from build123d import *

# Parameters (mm, degrees)
FILLET1_R     = 1
CHAMFER1_SIZE = 0.5
CHAMFER2_SIZE = 0.2


with BuildPart() as part:
    # Sketch1 → Revolve1 (revolve)
    with BuildSketch(Plane.XY, mode=Mode.PRIVATE) as revolve1_sk:
        Polygon((0, 0), (0, 8), (2.75, 8), (2.75, 6), (1.5, 6), (1.5, 0), align=None)
    revolve(revolve1_sk.sketch.rotate(Axis((0, 0, 0), (0, 1, 0)), 90), axis=Axis((0, 0, 0), (0, 1, 0)))

    # Fillet1
    fillet1_edges = [part.edges().sort_by_distance(p)[0] for p in [
        (0, 8, 2.75),
    ]]
    fillet(fillet1_edges, radius=FILLET1_R)

    # Chamfer1
    chamfer1_edges = [part.edges().sort_by_distance(p)[0] for p in [
        (0, 0, 1.5),
    ]]
    chamfer(chamfer1_edges, length=CHAMFER1_SIZE)

    # Chamfer2
    chamfer2_edges = [part.edges().sort_by_distance(p)[0] for p in [
        (0, 6, 2.75),
    ]]
    chamfer(chamfer2_edges, length=CHAMFER2_SIZE)


solid = part.part
Model file for the job. Use its own axes, mm. A direction names the side the tool comes from. Give positions to 0.01 mm unless a question says otherwise; leave off trailing zeros. Write each loop counter-clockwise with the first axis right and the second up, starting at its lowest first coordinate (ties: lowest second). Pieces come first, ordered by that corner, then holes. Notation, with made-up numbers: M 6,34.5 L 63,34.5 A11 ccw 63,40.5 Z; hole C -6.5,54.25 d10. An arc over 180 degrees is marked long. One line per item, written item: value. Start each with the question number.
Q1. Saw through at C-C, the plane y = 4. Write the cut outline in (x, z), plus the area to 3 significant figures.
Q2. Saw through at B-B, the plane z = 0. Write the cut outline in (x, y).
Q3. 3-axis set-ups, long thin cutter, end or side, ignore diameter. For faces 1 (the flat face through (0, 6, -2)), 2 (the flat face through (0, 0, 0)): which of +Z, -Z, +X, -X, +Y, -Y reach the whole face in a straight line?
Q4. Drop flat-ended pins along their axis: pin 1 Ø1.5 at (x, z) = (0.5, 0.5) entering from -Y; pin 2 Ø1.5 at (x, y) = (-0.5, 1) entering from +Z; pin 3 Ø2 at (y, z) = (2, 1) entering from -X. Give the stop position or say it passes through.
Q5. Saw through at A-A, the plane x = 0. Write the cut outline in (y, z), plus the area to 3 significant figures.
Q6. Probe probe 1 along Z at (x, y) = (-0.35, 5.5); probe 2 along Z at (x, y) = (-0.15, 6.25); probe 3 along X at (y, z) = (6.75, 0.35). List the from-to ranges inside material, lowest first. Write a range as [from, to].
Output values:
1. outline: C 0,0 d3
1. area: 7.07 mm²
2. outline: M -2.75,6.2 L -2.55,6 L -1.5,6 L -1.5,0.5 L -1,0 L 1,0 L 1.5,0.5 L 1.5,6 L 2.55,6 L 2.75,6.2 L 2.75,7 A1 ccw 1.75,8 L -1.75,8 A1 ccw -2.75,7 Z
3. face 1: -Y
3. face 2: +Z, -Z, +X, -X, -Y
4. pin 1: stops at y = 0
4. pin 2: stops at z = 1.5
4. pin 3: stops at x = -1.5
5. outline: M 0,-1 L 0.5,-1.5 L 6,-1.5 L 6,-2.55 L 6.2,-2.75 L 7,-2.75 A1 ccw 8,-1.75 L 8,1.75 A1 ccw 7,2.75 L 6.2,2.75 L 6,2.55 L 6,1.5 L 0.5,1.5 L 0,1 Z
5. area: 28.3 mm²
6. probe 1: z = [-1.46, 1.46]
6. probe 2: z = [-2.75, 2.75]
6. probe 3: x = [-2.73, 2.73]
